from build123d import *

# Parameters (mm, degrees)
F0_R          = 7.5
F2_DEPTH      = 254
F2_DEPTH_BACK = 254
F1_R          = 10
F3_DEPTH      = 203.2
F3_DEPTH_BACK = 203.2


with BuildPart() as f2:
    # F0 (on Right) → F2 (new body, two sides)
    with BuildSketch(Plane.YZ) as f2_sk:
        Circle(F0_R)
    extrude(amount=F2_DEPTH)
    extrude(f2_sk.sketch, amount=-F2_DEPTH_BACK)

    # F1 (on Right) → F3 (join, two sides)
    with BuildSketch(Plane.YZ) as f3_sk:
        Circle(F1_R)
    extrude(amount=F3_DEPTH)
    extrude(f3_sk.sketch, amount=-F3_DEPTH_BACK)


solid = f2.part
The model under review builds one solid part; all positions refer to its coordinate system, in mm. A direction names the side the tool comes from. Round coordinates to 2 decimals unless told otherwise and drop trailing zeros. Order: outer loops, then holes, each group sorted by start corner. A loop starts at its lowest first (then second) coordinate and runs counter-clockwise, first axis right, second up. Notation, with made-up numbers: (-2.75, 0.5) -> (54.25, 0.5) arc R22 cw to (54.25, 34.5) -> close; hole circle Ø8 at (-27.75, -35). An arc over 180 degrees is marked (long way). Return JSON: item names as keys, results as strings.
1. Insertion check: P1, Ø5, axis at x = 126.5, z = 5.5, coming from the -Y side; P2, Ø12, axis at x = 53.5, z = -2, coming from the -Y side; P3, Ø8, axis at x = -199, y = 4.5, coming from the -Z side; P4, Ø1.5, axis at x = 156.5, y = 2, coming from the -Z side. Each pin has a flat end and moves straight along its axis. Give the tip position at first contact, or say it passes through.
Answer block:
{"P1": "stops at y = -9.54", "P2": "stops at y = -10", "P3": "stops at z = -9.99", "P4": "stops at z = -9.92"}
2. For L1, parallel to Z at x = -115, y = -0.5; L2, parallel to Z at x = -107, y = -6.5; L3, parallel to X at y = -6.25, z = 6.5, list the stretches that pass through material, from the lowest coordinate up. Write a range as [from, to].
Answer block:
{"L1": "z = [-9.99, 9.99]", "L2": "z = [-7.6, 7.6]", "L3": "x = [-203.2, 203.2]"}
3. Take a section at C-C (x = 6.5). Write out the cut boundary in (y, z), then the cut area to 3 significant figures.
Answer block:
{"outline": "circle Ø20 at (0, 0)", "area": "314 mm²"}
4. For faces 1 (the face through (203.2, 4, 7)), 2 (the face through (254, 0, 0)), 3 (the face through (-203.2, 4, 7)), list the 3-axis set-ups (+Z, -Z, +X, -X, +Y, -Y) from which the entire face can be reached by the end or side of a thin tool; tool diameter is ignored.
Answer block:
{"face 1": "+X", "face 2": "+Z, -Z, +X, +Y, -Y", "face 3": "-X"}
5. Take a section at A-A (y = 0). Write out the cut boundary in (x, z).
Answer block:
{"outline": "(-254, -7.5) -> (-203.2, -7.5) -> (-203.2, -10) -> (203.2, -10) -> (203.2, -7.5) -> (254, -7.5) -> (254, 7.5) -> (203.2, 7.5) -> (203.2, 10) -> (-203.2, 10) -> (-203.2, 7.5) -> (-254, 7.5) -> close"}
